Geometry check sheet. Reference: the model listing, model coordinates, mm. Round coordinates to 2 decimals unless told otherwise and drop trailing zeros. Loops run counter-clockwise (first coordinate to the right, second up) from the corner with the lowest first, then second, coordinate; pieces in that order, holes last. Notation, with made-up numbers: (3.5, -9) - (51.5, -9) arc R32 cw to (51.5, 18) - close; hole circle Ø3 at (50, -16). An arc over 180 degrees is marked (long way). Answer as CSV lines item,"result". Start each with the question number.
1) Draft check along X on faces 1 (the flat face through (0, -3, 1)), 2 (the cylindrical face through (-0.085, 0.644, 1.197)). Enter one of: released by +X, released by -X, zero draft, split by the parting line, or undercut.
2) Thickness scan on line 1 along Y through (x, z) = (0, 1.2); line 2 along Z through (x, y) = (9.25, 7.5); line 3 along X through (y, z) = (-5, 0.9). Record the ranges inside material, lowest first.
3) Depth check by flat-ended pin: P1, Ø4, axis at x = -1.5, y = 6, coming from the +Z side. Enter the tip coordinate at first touch or a pass-through.
4) Cross-section at A-A on y = 0. Record the boundary of the cut face in (x, z), and give its area (3 significant figures).
from build123d import *

# Parameters (mm, degrees)
CYLINDER002_R     = 0.4
CYLINDER002_DEPTH = 0.6
CYLINDER001_R     = 0.65
CYLINDER001_DEPTH = 0.6
CHAMFER_SIZE      = 0.2
CYLINDER_R        = 0.4
CYLINDER_DEPTH    = 1
FILLET_R          = 0.8


with BuildPart() as cylinder002:
    # Cylinder002 → Cylinder002 (new body)
    with BuildSketch(Plane.XY.offset(1)):
        Circle(CYLINDER002_R)
    extrude(amount=CYLINDER002_DEPTH)


with BuildPart() as chamfer_body:
    # Cylinder001 → Cylinder001 (new body)
    with BuildSketch(Plane.XY.offset(1)):
        Circle(CYLINDER001_R)
    extrude(amount=CYLINDER001_DEPTH)

    # Cut001: cut Cylinder002
    add(cylinder002.part, mode=Mode.SUBTRACT)

    # Chamfer
    chamfer_edges = [chamfer_body.edges().sort_by_distance(p)[0] for p in [
        (-0.65, 0, 1.6),
    ]]
    chamfer(chamfer_edges, length=CHAMFER_SIZE)


with BuildPart() as cylinder:
    # Cylinder → Cylinder (new body)
    with BuildSketch(Plane.XY):
        Circle(CYLINDER_R)
    extrude(amount=CYLINDER_DEPTH)


with BuildPart() as fusion:
    # Cone → Cone (revolve)
    with BuildSketch(Plane.XZ):
        Polygon((0, 0), (14, 0), (13.8, 1), (0, 1), align=None)
    revolve(axis=Axis((0, 0, 0), (0, 0, 1)))

    # Cut: cut Cylinder
    add(cylinder.part, mode=Mode.SUBTRACT)

    # Fillet
    fillet_edges = [fusion.edges().sort_by_distance(p)[0] for p in [
        (-0.4, 0, 0),
    ]]
    fillet(fillet_edges, radius=FILLET_R)

    # Fusion: union Chamfer body
    add(chamfer_body.part)


solid = fusion.part
Answer block:
1,face 1,"zero draft"
1,face 2,"split by the parting line"
2,line 1,"y = -0.65 to -0.4, 0.4 to 0.65"
2,line 2,"z = 0 to 1"
2,line 3,"x = -12.88 to 12.88"
3,P1,"stops at z = 1"
4,outline,"(-14, 0) - (-1.2, 0) arc R0.8 ccw to (-0.4, 0.8) - (-0.4, 1.6) - (-0.45, 1.6) - (-0.65, 1.4) - (-0.65, 1) - (-13.8, 1) - close; (0.4, 0.8) arc R0.8 ccw to (1.2, 0) - (14, 0) - (13.8, 1) - (0.65, 1) - (0.65, 1.4) - (0.45, 1.6) - (0.4, 1.6) - close"
4,area,"27.0 mm^2"
